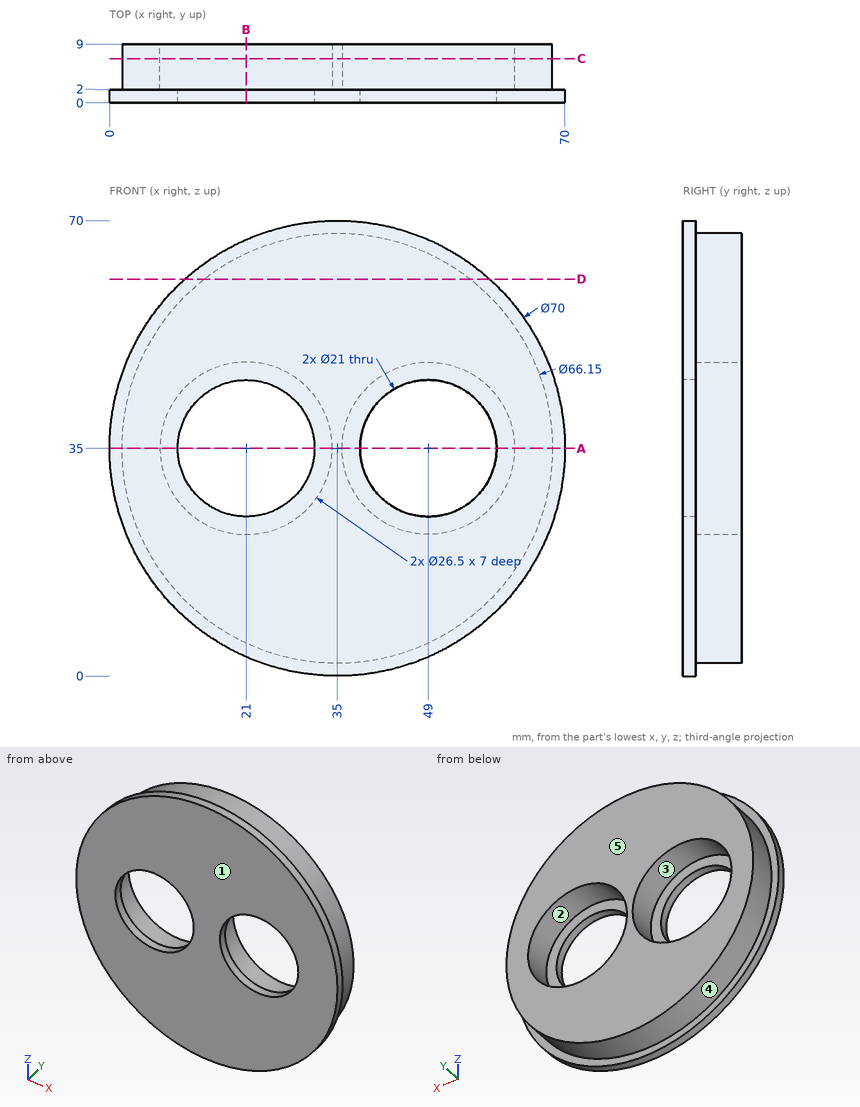
The figure shows three views and two pictorial views of one solid part (mm, origin at its lowest corner). Answer the questions. A direction names the side the tool comes from. Give positions to 0.01 mm unless a question says otherwise; leave off trailing zeros. Order: outer loops, then holes, each group sorted by start corner. A loop starts at its lowest first (then second) coordinate and runs counter-clockwise, first axis right, second up. Notation, with made-up numbers: (4, 66) - (45, 66) arc R13 ccw to (45, 90) - close; hole circle Ø10 at (-0.75, -12). An arc over 180 degrees is marked (long way). Answer as CSV lines item,"result".
Q1. A cutting plane is placed at C-C, the plane y = 6.75. Determine the outline of the cut face in (x, z) (3 decimals), and give its area (3 significant figures).
Answer key:
outline,"circle Ø66.15 at (35, 35); hole circle Ø26.5 at (21, 35); hole circle Ø26.5 at (49, 35)"
area,"2,330 mm^2"
Q2. A cutting plane is placed at B-B, the plane x = 21. Determine the outline of the cut face in (y, z).
Answer key:
outline,"(0, 2.92) - (2, 2.92) - (2, 5.03) - (9, 5.03) - (9, 21.75) - (2, 21.75) - (2, 24.5) - (0, 24.5) - close; (0, 45.5) - (2, 45.5) - (2, 48.25) - (9, 48.25) - (9, 64.97) - (2, 64.97) - (2, 67.08) - (0, 67.08) - close"
Q3. A cutting plane is placed at D-D, the plane z = 61. Determine the outline of the cut face in (x, y).
Answer key:
outline,"(11.57, 0) - (58.43, 0) - (58.43, 2) - (55.44, 2) - (55.44, 9) - (14.56, 9) - (14.56, 2) - (11.57, 2) - close"
Q4. Determine the mould class of the marked faces 3, 4 and 5 for opening direction X: pulls with the +X half, pulls with the -X half, needs draft (parallel to the pull), parting line crosses it, or undercut.
Answer key:
face 3,"undercut"
face 4,"parting line crosses it"
face 5,"needs draft"
Q5. Straight lines are drawn through the part: L1, parallel to X at y = 1, z = 26.5; L2, parallel to X at y = 8.25, z = 27.5; L3, parallel to Z at x = 28, y = 6.75. For each, find the intervals that lie inside material, in ascending order.
Answer key:
L1,"x = 1.05 to 14.84, 27.16 to 42.84, 55.16 to 68.95"
L2,"x = 2.79 to 10.08, 31.92 to 38.08, 59.92 to 67.21"
L3,"z = 2.67 to 23.75, 46.25 to 67.33"
Q6. Each of these flat-tipped pins is pushed along its axis until it touches: pin 1 Ø4 at (x, y) = (18.5, 8) entering from -Z; pin 2 Ø12 at (x, z) = (43, 43) entering from +Y; pin 3 Ø5 at (y, z) = (1, 54.5) entering from +X; pin 4 Ø8 at (x, z) = (42.5, 39) entering from +Y. Where does it stop, or does it pass through?
Answer key:
pin 1,"stops at z = 5.27"
pin 2,"stops at y = 9"
pin 3,"stops at x = 65.59"
pin 4,"stops at y = 2"
Q7. A cutting plane is placed at A-A, the plane z = 35. Determine the outline of the cut face in (x, y) (3 decimals).
Answer key:
outline,"(0, 0) - (10.5, 0) - (10.5, 2) - (7.75, 2) - (7.75, 9) - (1.925, 9) - (1.925, 2) - (0, 2) - close; (31.5, 0) - (38.5, 0) - (38.5, 2) - (35.75, 2) - (35.75, 9) - (34.25, 9) - (34.25, 2) - (31.5, 2) - close; (59.5, 0) - (70, 0) - (70, 2) - (68.075, 2) - (68.075, 9) - (62.25, 9) - (62.25, 2) - (59.5, 2) - close"
Q8. Which of the six approach directions +Z, -Z, +X, -X, +Y, -Y give full straight-line access (tool end or side, diameter ignored) to the marked faces 1 and 2?
Answer key:
face 1,"+Z, -Z, +X, -X, -Y"
face 2,"+Y"
